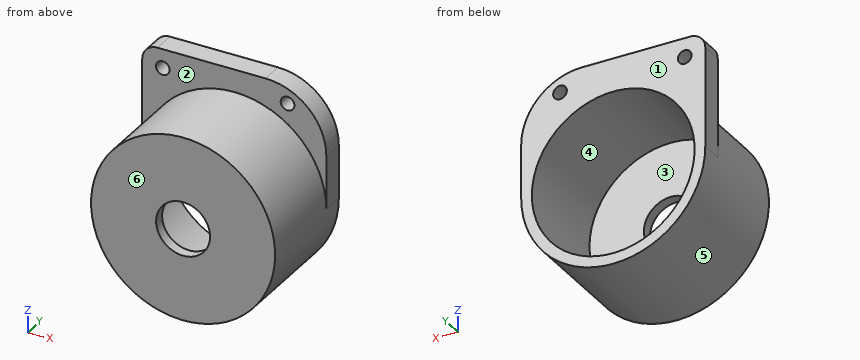
```python
from build123d import *

# Parameters (mm, degrees)
SKETCH_1_R          = 60.5
EXTRUDE_1_DEPTH     = 7
SKETCH_2_R          = 60.5
SKETCH_2_R_2        = 53.5
EXTRUDE_2_DEPTH     = 67
SKETCH_3_R          = 17.75
CUT_EXTRUDE_1_DEPTH = 54
SKETCH_6_R          = 4.5
EXTRUDE_3_DEPTH     = 14.5


with BuildPart() as part:
    # Эскиз1 → Бобышка-Вытянуть1 (new body)
    with BuildSketch(Plane(origin=(0, 0, 0), x_dir=(1, 0, 0), z_dir=(0, 1, 0))):
        Circle(SKETCH_1_R)
    extrude(amount=EXTRUDE_1_DEPTH)

    # Эскиз2 → Бобышка-Вытянуть2 (add)
    with BuildSketch(Plane(origin=(0, 7, 0), x_dir=(1, 0, 0), z_dir=(0, 1, 0))):
        Circle(SKETCH_2_R)
        Circle(SKETCH_2_R_2, mode=Mode.SUBTRACT)
    extrude(amount=EXTRUDE_2_DEPTH)

    # Эскиз3 → Вырез-Вытянуть1 (cut)
    with BuildSketch(Plane(origin=(0, 7, 0), x_dir=(1, 0, 0), z_dir=(0, 1, 0))):
        Circle(SKETCH_3_R)
    extrude(amount=-CUT_EXTRUDE_1_DEPTH, mode=Mode.SUBTRACT)

    # Эскиз6 → Бобышка-Вытянуть3 (add)
    with BuildSketch(Plane(origin=(0, 74, 0), x_dir=(1, 0, 0), z_dir=(0, 1, 0))):
        with BuildLine():
            ThreePointArc((60.5, 0), (0, -60.5), (-60.5, 0))
            Line((-60.5, 0), (-60.5, -65.387945457))
            ThreePointArc((-60.5, -65.387945457), (-57.571067812, -72.459013269), (-50.5, -75.387945457))
            Line((-50.5, -75.387945457), (20.5, -75.387945457))
            ThreePointArc((20.5, -75.387945457), (48.784271247, -63.672216704), (60.5, -35.387945457))
            Line((60.5, -35.387945457), (60.5, 0))
        make_face()
        with Locations((-47, -62.890262607)):
            Circle(SKETCH_6_R, mode=Mode.SUBTRACT)
        with BuildLine():
            ThreePointArc((39.5, -62.890262607), (35, -67.390262607), (30.5, -62.890262607))
            ThreePointArc((30.5, -62.890262607), (35, -58.390262607), (39.5, -62.890262607))
        make_face(mode=Mode.SUBTRACT)
    extrude(amount=-EXTRUDE_3_DEPTH)


solid = part.part
```
Read the model definition and answer for the solid it produces. Units are mm, in the model's axes. Face numbers are marked on the shaded views. A direction names the side the tool comes from. Coordinates: 2 decimals unless noted, no trailing zeros. Loops run counter-clockwise (first coordinate to the right, second up) from the corner with the lowest first, then second, coordinate; pieces in that order, holes last. Notation, with made-up numbers: (-27, -10) -> (25, -10) arc R8 cw to (25, -1) -> close; hole circle Ø9 at (83.5, 50.5). An arc over 180 degrees is marked (long way). Return JSON: item names as keys, results as strings.
Item 1: For a pull along X with two mould halves and no side action, classify the marked faces 4, 5 and 6 as +X half, -X half, draft (parallel to the pull), parting line (faces both ways), or undercut.
Answers:
{"face 4": "undercut", "face 5": "parting line", "face 6": "draft"}
Item 2: Find the intervals of material crossed by probe 1 along Z at (x, y) = (-1, 61); probe 2 along Z at (x, y) = (0, 2); probe 3 along Z at (x, y) = (-47, 64), in increasing order.
Answers:
{"probe 1": "z = -60.49 to -53.49, 53.49 to 75.39", "probe 2": "z = -60.5 to -17.75, 17.75 to 60.5", "probe 3": "z = -38.1 to -25.56, 25.56 to 58.39, 67.39 to 75.39"}
Item 3: Find section D-D (z = -22). Determine the outline of the cut face in (x, y).
Answers:
{"outline": "(-56.36, 0) -> (56.36, 0) -> (56.36, 74) -> (48.77, 74) -> (48.77, 7) -> (-48.77, 7) -> (-48.77, 74) -> (-56.36, 74) -> close"}
Item 4: Find section C-C (x = 35). Determine the outline of the cut face in (y, z), plus the area to 3 significant figures.
Answers:
{"outline": "(0, -49.35) -> (74, -49.35) -> (74, -40.46) -> (7, -40.46) -> (7, 40.46) -> (74, 40.46) -> (74, 58.39) -> (59.5, 58.39) -> (59.5, 49.35) -> (0, 49.35) -> close; (59.5, 67.39) -> (74, 67.39) -> (74, 72.67) -> (59.5, 72.67) -> close", "area": "2,090 mm2"}
Item 5: Find section B-B (y = 44). Determine the outline of the cut face in (x, z).
Answers:
{"outline": "circle Ø121 at (0, 0); hole circle Ø107 at (0, 0)"}
Item 6: Flat-ended cylindrical pins translate along their axes: P1, Ø8, axis at y = 33.5, z = 11, coming from the +X side; P2, Ø12, axis at x = 0.5, y = 39, coming from the +Z side; P3, Ø2, axis at y = 42.5, z = 16.5, coming from the -X side. Find the tip coordinate at first contact, or state that the pin passes through.
Answers:
{"P1": "stops at x = 60.09", "P2": "stops at z = 60.5", "P3": "stops at x = -58.48"}
Item 7: Find section A-A (x = 0). Determine the outline of the cut face in (y, z).
Answers:
{"outline": "(0, -60.5) -> (74, -60.5) -> (74, -53.5) -> (7, -53.5) -> (7, -17.75) -> (0, -17.75) -> close; (0, 17.75) -> (7, 17.75) -> (7, 53.5) -> (74, 53.5) -> (74, 75.39) -> (59.5, 75.39) -> (59.5, 60.5) -> (0, 60.5) -> close"}
Item 8: For the marked faces 1, 2 and 3, determine the directions among +Z, -Z, +X, -X, +Y, -Y from which every point of the face is accessible in a straight line to the end or side of a thin tool.
Answers:
{"face 1": "+Z, -Z, +X, -X, +Y", "face 2": "+Z, -Y", "face 3": "+Y"}
